Can you work these out from the model? Positions are in its coordinate system, mm. A direction names the side the tool comes from. Round coordinates to 2 decimals unless told otherwise and drop trailing zeros. Write each loop counter-clockwise with the first axis right and the second up, starting at its lowest first coordinate (ties: lowest second). Pieces come first, ordered by that corner, then holes. Notation, with made-up numbers: (8.25, 45.25) -> (26.25, 45.25) arc R23 cw to (26.25, 82.25) -> close; hole circle Ø10 at (26.25, -3.75). An arc over 180 degrees is marked (long way). Use CSV: the item, a comma, the result in double quotes.
```python
from build123d import *

# Parameters (mm, degrees)
SKETCH003_W     = 93
SKETCH003_H     = 70
PAD003_DEPTH    = 1.6
SKETCH_W        = 88
SKETCH_H        = 53.7
PAD_DEPTH       = 8.4
SKETCH004_W     = 70
SKETCH004_H     = 38.8
POCKET_DEPTH    = 2
SKETCH005_R     = 1.5
POCKET001_DEPTH = 1.601
SKETCH006_W     = 54
SKETCH006_H     = 5
PAD004_DEPTH    = 10
SKETCH007_W     = 54
SKETCH007_H     = 20
PAD005_DEPTH    = 1.6
SKETCH008_W     = 20
SKETCH008_H     = 15
PAD006_DEPTH    = 3


with BuildPart() as part:
    # Sketch003 → Pad003 (new body)
    with BuildSketch(Plane.XY):
        Rectangle(SKETCH003_W, SKETCH003_H)
    extrude(amount=PAD003_DEPTH)

    # Sketch (on DatumPlane) → Pad (join)
    with BuildSketch(Plane.XY.offset(1.6)):
        Rectangle(SKETCH_W, SKETCH_H)
    extrude(amount=PAD_DEPTH)

    # Sketch004 (on DatumPlane) → Pocket (cut)
    with BuildSketch(Plane.XY.offset(10)):
        Rectangle(SKETCH004_W, SKETCH004_H)
    extrude(amount=-POCKET_DEPTH, mode=Mode.SUBTRACT)

    # Sketch005 (on DatumPlane) → Pocket001 (cut, through all)
    with BuildSketch(Plane.XY.offset(1.6)):
        with Locations((-44, 32.5)):
            Circle(SKETCH005_R)
        with Locations((44, 32.5)):
            Circle(SKETCH005_R)
        with Locations((-44, -32.5)):
            Circle(SKETCH005_R)
        with Locations((44, -32.5)):
            Circle(SKETCH005_R)
    extrude(amount=-POCKET001_DEPTH, mode=Mode.SUBTRACT)

    # Sketch006 (on DatumPlane) → Pad004 (join)
    with BuildSketch(Plane(origin=(0, 0, 0), x_dir=(1, 0, 0), z_dir=(0, 0, -1))):
        with Locations((10, -32.5)):
            Rectangle(SKETCH006_W, SKETCH006_H)
    extrude(amount=PAD004_DEPTH)

    # Sketch007 (on DatumPlane) → Pad005 (join)
    with BuildSketch(Plane(origin=(0, 0, -4), x_dir=(1, 0, 0), z_dir=(0, 0, -1))):
        with Locations((10, -25)):
            Rectangle(SKETCH007_W, SKETCH007_H)
    extrude(amount=PAD005_DEPTH)

    # Sketch008 (on DatumPlane) → Pad006 (join)
    with BuildSketch(Plane(origin=(0, 0, -4), x_dir=(1, 0, 0), z_dir=(0, 0, -1))):
        with Locations((-20, -27.5)):
            Rectangle(SKETCH008_W, SKETCH008_H)
    extrude(amount=-PAD006_DEPTH)


solid = part.part
```
Q1. Suppose I cut it at C-C (y = 32.5). Write out the boundary of the cut face in (x, z), and give its area (3 significant figures).
Resolved:
outline,"(-46.5, 0) -> (-45.5, 0) -> (-45.5, 1.6) -> (-46.5, 1.6) -> close; (-42.5, 0) -> (-17, 0) -> (-17, -1) -> (-30, -1) -> (-30, -4) -> (-17, -4) -> (-17, -10) -> (37, -10) -> (37, 0) -> (42.5, 0) -> (42.5, 1.6) -> (-42.5, 1.6) -> close; (45.5, 0) -> (46.5, 0) -> (46.5, 1.6) -> (45.5, 1.6) -> close"
area,"718 mm^2"
Q2. Please list where these lines run through material, in increasing order: probe 1 along Y at (x, z) = (-44, 1.1); probe 2 along Z at (x, y) = (31, 27); probe 3 along Z at (x, y) = (6, 17.5).
Resolved:
probe 1,"y = -35 to -34, -31 to 31, 34 to 35"
probe 2,"z = -5.6 to -4, 0 to 1.6"
probe 3,"z = -5.6 to -4, 0 to 8"
Q3. Suppose I cut it at B-B (x = -14). Write out the boundary of the cut face in (y, z), and give its area (3 significant figures).
Resolved:
outline,"(-35, 0) -> (30, 0) -> (30, -1) -> (20, -1) -> (20, -4) -> (15, -4) -> (15, -5.6) -> (30, -5.6) -> (30, -10) -> (35, -10) -> (35, 1.6) -> (26.85, 1.6) -> (26.85, 10) -> (19.4, 10) -> (19.4, 8) -> (-19.4, 8) -> (-19.4, 10) -> (-26.85, 10) -> (-26.85, 1.6) -> (-35, 1.6) -> close"
area,"589 mm^2"
Q4. On a 3-axis mill with a long thin cutter (end or side, diameter ignored), from which of +Z, -Z, +X, -X, +Y, -Y can I reach the whole of each face in a straight line? I mean faces 4 (the face through (35, 0, 9)), 5 (the face through (10, 22, -5.6)), 6 (the face through (-24, 27, -4)), 7 (the face through (44, 0, 6)), 8 (the face through (-20, 27, -1)). Say none if no direction works.
Resolved:
face 4,"+Z"
face 5,"-Z, +X, -X, -Y"
face 6,"-Z, -X, +Y, -Y"
face 7,"+Z, +X, +Y, -Y"
face 8,"-X, -Y"
Q5. Suppose I cut it at D-D (z = -7.75). Write out the boundary of the cut face in (x, y), and give its area (3 significant figures).
Resolved:
outline,"(-17, 30) -> (37, 30) -> (37, 35) -> (-17, 35) -> close"
area,"270 mm^2"
Q6. Will these pins go through, and if not, where does the flat tip stop? P1, Ø5, axis at x = -44, y = 32.5, coming from the -Z side; P2, Ø1.5, axis at y = 24, z = -2.5, coming from the +X side; P3, Ø3.5, axis at x = -23.5, z = -3, coming from the -Y side; P4, Ø2.5, axis at x = 44, y = -32.5, coming from the +Z side.
Resolved:
P1,"stops at z = 0"
P2,"stops at x = -10"
P3,"stops at y = 20"
P4,"passes through"
Q7. Suppose I cut it at A-A (y = -32.5). Write out the boundary of the cut face in (x, z).
Resolved:
outline,"(-46.5, 0) -> (-45.5, 0) -> (-45.5, 1.6) -> (-46.5, 1.6) -> close; (-42.5, 0) -> (42.5, 0) -> (42.5, 1.6) -> (-42.5, 1.6) -> close; (45.5, 0) -> (46.5, 0) -> (46.5, 1.6) -> (45.5, 1.6) -> close"
Q8. If we mould it in two halves opening along Y, with no side actions, what happens to faces 1 (the face through (-44, 0, 6)), 2 (the face through (-1, 26.85, 6)), 3 (the face through (42.8, 31.6, 0.8))? For each: released by +Y, released by -Y, zero draft, split by the parting line, or undercut.
Resolved:
face 1,"zero draft"
face 2,"released by +Y"
face 3,"undercut"
